Could you check a few things on this model? Use its own coordinates, in mm. A direction names the side the tool comes from. Round coordinates to 2 decimals unless told otherwise and drop trailing zeros. Loops run counter-clockwise (first coordinate to the right, second up) from the corner with the lowest first, then second, coordinate; pieces in that order, holes last. Notation, with made-up numbers: (23, 26) -> (71, 26) arc R13 ccw to (71, 36) -> close; hole circle Ø4 at (-32.75, 72.25). An arc over 180 degrees is marked (long way). Write each question's results on one line, items separated by ' | '.
from build123d import *

# Parameters (mm, degrees)
PAD074_DEPTH            = 18.9
PAD078_DEPTH            = 7.8
FILLET020_R             = 2
BODY067_ROLL_ANGLE      = 180
BODY067_PLACEMENT_ANGLE = 90


with BuildPart() as part:
    # Sketch124 → Pad074 (new body)
    with BuildSketch(Plane.XY):
        with BuildLine():
            Line((-30, 30), (-30, -30))
            Line((-30, -30), (30, -30))
            Line((30, -30), (30, -16.2))
            ThreePointArc((30, -16.2), (28.828427, -13.371573), (26, -12.2))
            Line((26, -12.2), (-12.2, -12.2))
            Line((-12.2, -12.2), (-12.2, 26))
            ThreePointArc((-12.2, 26), (-13.371573, 28.828427), (-16.2, 30))
            Line((-16.2, 30), (-30, 30))
        make_face()
        with BuildLine():
            Line((-28.4, 28.4), (-16.2, 28.4))
            ThreePointArc((-13.8, 26), (-14.502944, 27.697056), (-16.2, 28.4))
            Line((-13.8, 26), (-13.8, -13.8))
            Line((-13.8, -13.8), (26, -13.8))
            ThreePointArc((28.4, -16.2), (27.697056, -14.502944), (26, -13.8))
            Line((28.4, -16.2), (28.4, -28.4))
            Line((28.4, -28.4), (-28.4, -28.4))
            Line((-28.4, -28.4), (-28.4, 28.4))
        make_face(mode=Mode.SUBTRACT)
    extrude(amount=PAD074_DEPTH)

    # Sketch128 → Pad078 (join)
    with BuildSketch(Plane.XY):
        Polygon((-13.8, 29.2), (-13.8, -13.8), (29.2, -13.8), align=None)
    extrude(amount=PAD078_DEPTH)

    # Fillet020
    fillet020_edges = [part.edges().sort_by_distance(p)[0] for p in [
        (7.7, 7.7, 7.8),
    ]]
    fillet(fillet020_edges, radius=FILLET020_R)


with BuildPart() as part_1:
    # Body067 roll: moved
    add(part.part.rotate(Axis((0, 0, 0), (1, 0, 0)), BODY067_ROLL_ANGLE))


with BuildPart() as part_2:
    # Body067 placement: moved
    add(part_1.part.moved(Location((-115.5, -115.5, 78.1))).rotate(Axis((-115.5, -115.5, 78.1), (0, 0, 1)), BODY067_PLACEMENT_ANGLE))


solid = part_2.part
1) I want a section at C-C, the plane z = 73. Write out the boundary of the cut face in (x, y), plus the area to 3 significant figures.
Model answer:
outline: (-145.5, -145.5) -> (-85.5, -145.5) -> (-85.5, -131.7) arc R4 ccw to (-87.1, -128.5) -> (-128.5, -87.1) arc R4 ccw to (-131.7, -85.5) -> (-145.5, -85.5) -> close; hole (-143.9, -143.9) -> (-87.1, -143.9) -> (-87.1, -131.7) arc R2.4 ccw to (-89.5, -129.3) -> (-129.3, -129.3) -> (-129.3, -89.5) arc R2.4 ccw to (-131.7, -87.1) -> (-143.9, -87.1) -> close | area: 1,160 mm2
2) I'm going to push flat-ended pins straight in: pin 1 (5 mm diameter, centred on y = -111, z = 61, fed in from +X); pin 2 (11 mm diameter, centred on x = -100.5, y = -111, fed in from -Z); pin 3 (5 mm diameter, centred on y = -97, z = 76, fed in from +X). Where does each tip first touch, or does it pass through?
Model answer:
pin 1: stops at x = -127.7 | pin 2: stops at z = 70.3 | pin 3: stops at x = -116.1
3) I need wall thicknesses on line 1 (Y direction, x = -92, z = 60.5); line 2 (X direction, y = -134, z = 65.5). Which ranges of each line are inside material? Lowest first, please.
Model answer:
line 1: y = -145.5 to -143.9, -129.3 to -127.7 | line 2: x = -145.5 to -143.9, -87.1 to -85.5
4) I want a section at A-A, the plane z = 62.5. Write out the boundary of the cut face in (x, y), plus the area to 3 significant figures.
Model answer:
outline: (-145.5, -145.5) -> (-85.5, -145.5) -> (-85.5, -131.7) arc R4 ccw to (-89.5, -127.7) -> (-127.7, -127.7) -> (-127.7, -89.5) arc R4 ccw to (-131.7, -85.5) -> (-145.5, -85.5) -> close; hole (-143.9, -143.9) -> (-87.1, -143.9) -> (-87.1, -131.7) arc R2.4 ccw to (-89.5, -129.3) -> (-129.3, -129.3) -> (-129.3, -89.5) arc R2.4 ccw to (-131.7, -87.1) -> (-143.9, -87.1) -> close | area: 369 mm2
5) For faces 1 (the flat face through (-85.5, -139, 69)), 2 (the flat face through (-109, -129.3, 69)), 3 (the flat face through (-109, -127.7, 65)), which set-ups out of +Z, -Z, +X, -X, +Y, -Y let a thin tool reach every point of the face, with its end or its side?
Model answer:
face 1: +Z, -Z, +X, +Y, -Y | face 2: +Z, -Z | face 3: -Z, +X, +Y
6) I want a section at B-B, the plane y = -130.5. Write out the boundary of the cut face in (x, z).
Model answer:
outline: (-145.5, 59.2) -> (-143.9, 59.2) -> (-143.9, 78.1) -> (-145.5, 78.1) -> close; (-87.42, 59.2) -> (-85.68, 59.2) -> (-85.68, 78.1) -> (-87.42, 78.1) -> close
